The figure shows three views and two pictorial views of one solid part (mm, origin at its lowest corner). Answer the questions. Coordinates: 2 decimals unless noted, no trailing zeros. Loops run counter-clockwise (first coordinate to the right, second up) from the corner with the lowest first, then second, coordinate; pieces in that order, holes last. Notation, with made-up numbers: M -6,65.5 L 34,65.5 A17 cw 34,94.5 Z; hole C 88.25,56 d8. An arc over 180 degrees is marked long. Return JSON: item names as keys, results as strings. Group by question number.
1. Given P1, Ø3, axis at y = 1.5, z = 23, coming from the +X side; P2, Ø6, axis at x = 3.5, z = 32, coming from the +Y side; P3, Ø4, axis at x = 6.5, y = 6.5, coming from the +Z side; P4, Ø8, axis at x = 9.5, y = 6, coming from the -Z side, each flat-ended and moving along its own axis, determine where each tip first touches the part or whether it passes through.
2. Section C-C (x = 1.75) is taken. Write down the section's boundary in (y, z).
3. The mould has two halves that part along Y. Classify the marked faces 1 and 2: pulls with the +Y half, pulls with the -Y half, needs draft (parallel to the pull), parting line crosses it, or undercut.
4. Straight lines are drawn through the part: L1, parallel to Y at x = 11, z = 30; L2, parallel to X at y = 2.75, z = 37.5; L3, parallel to Y at x = 10.75, z = 34.5. For each, find the intervals that lie inside material, in ascending order. Write a range as from..to.
5. Section D-D (y = 2.5) is taken. Write down the section's boundary in (x, z), then the cut area to 3 significant figures.
6. Section A-A (x = 10) is taken. Write down the section's boundary in (y, z), then the cut area to 3 significant figures.
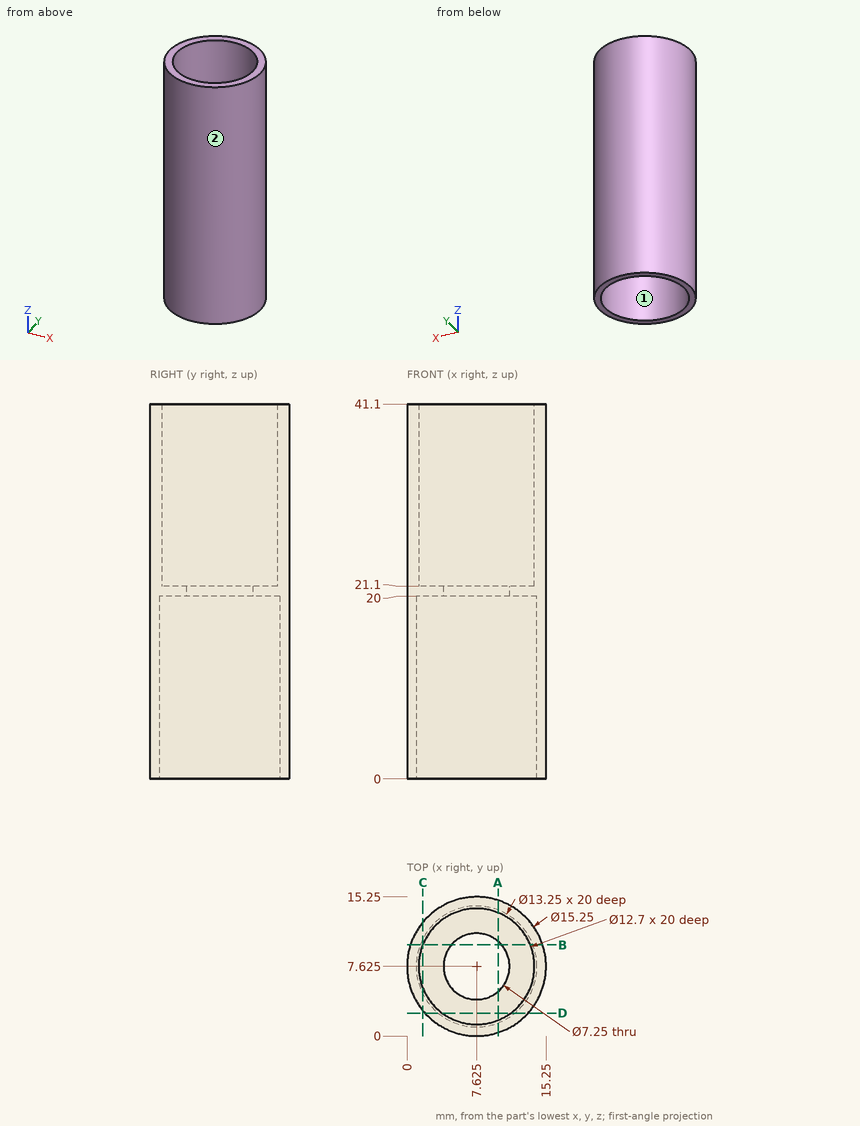
Worked out:
{
 "1": {"P1": "x = 13.69", "P2": "y = 15.17", "P3": "through", "P4": "z = 20"},
 "2": {"outline": "M 2.76,0 L 4.56,0 L 4.56,20 L 10.69,20 L 10.69,0 L 12.49,0 L 12.49,41.1 L 10.03,41.1 L 10.03,21.1 L 5.22,21.1 L 5.22,41.1 L 2.76,41.1 Z"},
 "3": {"face 1": "undercut", "face 2": "parting line crosses it"},
 "4": {"L1": "0.79..2.25, 13..14.46", "L2": "1.76..3.56, 11.69..13.49", "L3": "0.67..2.1, 13.15..14.58"},
 "5": {"outline": "M 1.98,0 L 3.43,0 L 3.43,20 L 11.82,20 L 11.82,0 L 13.27,0 L 13.27,41.1 L 11.37,41.1 L 11.37,21.1 L 3.88,21.1 L 3.88,41.1 L 1.98,41.1 Z", "area": "146 mm^2"},
 "6": {"outline": "M 0.38,0 L 1.44,0 L 1.44,20 L 4.89,20 L 4.89,21.1 L 1.74,21.1 L 1.74,41.1 L 0.38,41.1 Z; M 10.36,20 L 13.81,20 L 13.81,0 L 14.87,0 L 14.87,41.1 L 13.51,41.1 L 13.51,21.1 L 10.36,21.1 Z", "area": "107 mm^2"}
}
